Model file for the job. Use its own axes, mm. Face numbers are marked on the shaded views. A direction names the side the tool comes from. Coordinates: 2 decimals unless noted, no trailing zeros. Order: outer loops, then holes, each group sorted by start corner. A loop starts at its lowest first (then second) coordinate and runs counter-clockwise, first axis right, second up.
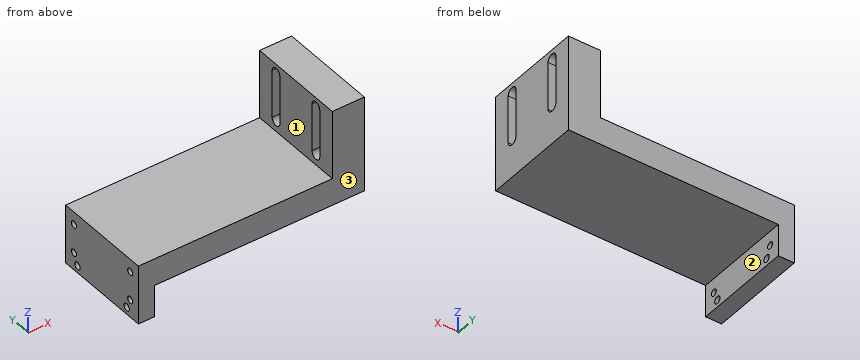
from build123d import *

# Parameters (mm, degrees)
SKETCH_1_W             = 141.2
SKETCH_1_H             = 62
EXTRUDE_1_DEPTH        = 80
SKETCH_2_W             = 131.2
SKETCH_2_H             = 20
SKETCH_2_W_2           = 121.2
SKETCH_2_H_2           = 43
CUT_EXTRUDE_1_DEPTH    = 174.728063363
CUT_EXTRUDE_2_DEPTH    = 70
SKETCH_4_R             = 2.25
CUT_EXTRUDE_3_DEPTH    = 166.702866602
HOLE_WIZARD_M5_1_D     = 4.2
HOLE_WIZARD_M5_1_DEPTH = 12.4
HOLE_WIZARD_M5_1_TIP   = 1.2618073


with BuildPart() as part:
    # 草图1 → 凸台-拉伸1 (new body)
    with BuildSketch(Plane.XY):
        with Locations((70.6, 31)):
            Rectangle(SKETCH_1_W, SKETCH_1_H)
    extrude(amount=EXTRUDE_1_DEPTH)

    # 草图2 → 切除-拉伸1 (cut, through all)
    with BuildSketch(Plane.XZ):
        with Locations((75.6, 10)):
            Rectangle(SKETCH_2_W, SKETCH_2_H)
        with Locations((60.6, 58.5)):
            Rectangle(SKETCH_2_W_2, SKETCH_2_H_2)
    extrude(amount=-CUT_EXTRUDE_1_DEPTH, mode=Mode.SUBTRACT)

    # 草图3 → 切除-拉伸2 (cut)
    with BuildSketch(Plane.ZY.offset(-121.2)):
        with BuildLine():
            Line((44, 17.3), (74, 17.3))
            ThreePointArc((74, 17.3), (77.3, 14), (74, 10.7))
            Line((74, 10.7), (44, 10.7))
            ThreePointArc((44, 10.7), (40.7, 14), (44, 17.3))
        make_face()
        with BuildLine():
            Line((44, 44.7), (74, 44.7))
            ThreePointArc((74, 44.7), (77.3, 48), (74, 51.3))
            Line((74, 51.3), (44, 51.3))
            ThreePointArc((44, 51.3), (40.7, 48), (44, 44.7))
        make_face()
    extrude(amount=-CUT_EXTRUDE_2_DEPTH, mode=Mode.SUBTRACT)

    # 草图4 → 切除-拉伸3 (cut, through all)
    with BuildSketch(Plane(origin=(10, 0, 0), x_dir=(0, 0, -1), z_dir=(1, 0, 0))):
        with Locations(Location((-4.5, 10, 0), (0, 0, 180))):
            Circle(SKETCH_4_R)
        with Locations((-4.5, 52)):
            Circle(SKETCH_4_R)
    extrude(amount=-CUT_EXTRUDE_3_DEPTH, mode=Mode.SUBTRACT)

    # M5 螺纹孔1
    with Locations(Plane.ZY):
        with Locations((29, 7), (11, 7), (11, 55), (29, 55)):
            Hole(HOLE_WIZARD_M5_1_D / 2, depth=HOLE_WIZARD_M5_1_DEPTH)
            with Locations((0, 0, -(HOLE_WIZARD_M5_1_DEPTH + HOLE_WIZARD_M5_1_TIP / 2))):  # 118° drill point
                Cone(0, HOLE_WIZARD_M5_1_D / 2, HOLE_WIZARD_M5_1_TIP, mode=Mode.SUBTRACT)


solid = part.part
Q1. Probe line 1 (Y direction, x = 4.75, z = 4.5); line 2 (Y direction, x = 3, z = 29); line 3 (X direction, y = 35.5, z = 68). List the from-to ranges inside material, lowest first.
Established:
line 1: y = 0 to 7.75, 12.25 to 49.75, 54.25 to 62
line 2: y = 0 to 4.9, 9.1 to 52.9, 57.1 to 62
line 3: x = 121.2 to 141.2
Q2. Cut at B-B, the plane z = 4.5. List the corners of the cut face in (x, y).
Established:
outline: (0, 0) - (10, 0) - (10, 7.75) - (0, 7.75) - close; (0, 12.25) - (10, 12.25) - (10, 49.75) - (0, 49.75) - close; (0, 54.25) - (10, 54.25) - (10, 62) - (0, 62) - close
Q3. Cut at A-A, the plane y = 48. List the corners of the cut face in (x, z).
Established:
outline: (0, 0) - (10, 0) - (10, 20) - (141.2, 20) - (141.2, 40.7) - (121.2, 40.7) - (121.2, 37) - (0, 37) - close; (121.2, 77.3) - (141.2, 77.3) - (141.2, 80) - (121.2, 80) - close
Q4. Drop flat-ended pins along their axis: P1, Ø4, axis at x = 48.5, y = 54.5, coming from the -Z side; P2, Ø2.5, axis at y = 7, z = 11, coming from the +X side; P3, Ø5, axis at y = 55, z = 11, coming from the +X side; P4, Ø3, axis at x = 48, y = 47, coming from the +Z side. Give the stop position or say it passes through.
Established:
P1: stops at z = 20
P2: passes through
P3: stops at x = 10
P4: stops at z = 37
Q5. Cut at D-D, the plane x = 29.5. List the corners of the cut face in (y, z).
Established:
outline: (0, 20) - (62, 20) - (62, 37) - (0, 37) - close
Q6. Which spindle directions (+Z, -Z, +X, -X, +Y, -Y) get a long thin tool onto all of the face, cutting with end or side? Do the marked faces 1, 2 and 3. Say none if no direction does.
Established:
face 1: +Z, -X, +Y, -Y
face 2: -Z, +X, +Y, -Y
face 3: +Z, -Z, +X, -X, -Y
Q7. Cut at C-C, the plane z = 56. List the corners of the cut face in (x, y), plus the area to 3 significant figures.
Established:
outline: (121.2, 0) - (141.2, 0) - (141.2, 10.7) - (121.2, 10.7) - close; (121.2, 17.3) - (141.2, 17.3) - (141.2, 44.7) - (121.2, 44.7) - close; (121.2, 51.3) - (141.2, 51.3) - (141.2, 62) - (121.2, 62) - close
area: 976 mm2
